```python
from build123d import *

# Parameters (mm, degrees)
F0_R     = 6
F1_DEPTH = 32
F3_W     = 12
F3_H     = 45
F4_DEPTH = 55.801
F5_R     = 4


with BuildPart() as f1:
    # F0 (on Front) → F1 (new body)
    with BuildSketch(Plane.XZ):
        with BuildLine():
            Line((15, -27.838539), (15, 58.161461))
            ThreePointArc((15, 58.161461), (-11.61895, 67.648294), (3, 43.464522))
            Line((3, 43.464522), (3, -27.838539))
            Line((3, -27.838539), (15, -27.838539))
        make_face()
        with Locations((0, 58.161461)):
            Circle(F0_R, mode=Mode.SUBTRACT)
    extrude(amount=F1_DEPTH)

    # F3 (on offset) → F4 (cut, through all)
    with BuildSketch(Plane.YZ.offset(-40.8)):
        with BuildLine():
            Line((0, -27.838539), (0, -11.838539))
            ThreePointArc((0, -11.838539), (-4.686292, -23.152248), (-16, -27.838539))
            Line((-16, -27.838539), (0, -27.838539))
        make_face()
        with BuildLine():
            Line((-32, -27.838539), (-16, -27.838539))
            ThreePointArc((-16, -27.838539), (-27.313708, -23.152248), (-32, -11.838539))
            Line((-32, -11.838539), (-32, -27.838539))
        make_face()
        with BuildLine():
            Line((-10, -11.838539), (-10, 13.161461))
            ThreePointArc((-10, 13.161461), (-16, 19.161461), (-22, 13.161461))
            Line((-22, 13.161461), (-22, -11.838539))
            ThreePointArc((-22, -11.838539), (-16, -17.838539), (-10, -11.838539))
        make_face()
        with Locations((-16, 50.661461)):
            Rectangle(F3_W, F3_H)
    extrude(amount=F4_DEPTH, mode=Mode.SUBTRACT)

    # F5
    f5_edges = [f1.edges().sort_by_distance(p)[0] for p in [
        (3, -5, 43.464522),
        (3, -27, 43.464522),
    ]]
    fillet(f5_edges, radius=F5_R)


solid = f1.part
```
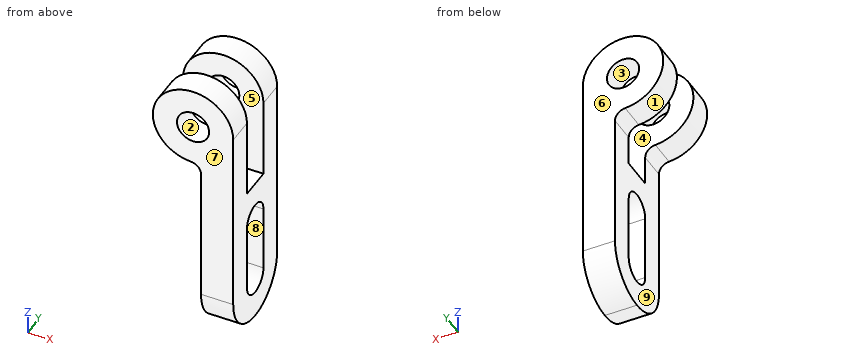
Can you work these out from the model? Positions are in its coordinate system, mm. Face numbers are marked on the shaded views. A direction names the side the tool comes from. Coordinates: 2 decimals unless noted, no trailing zeros. Write each loop counter-clockwise with the first axis right and the second up, starting at its lowest first coordinate (ties: lowest second). Pieces come first, ordered by that corner, then holes. Notation, with made-up numbers: M 86,-34 L 144,-34 A12 ccw 144,-28 Z; hole C -2.75,36.25 d6. An arc over 180 degrees is marked long. Write item = value, one per line. Start each with the question number.
Q1. If I drill on L1, parallel to Y at x = 2.5, z = 44; L2, parallel to X at y = -29, z = 1; L3, parallel to Z at x = 0, y = -2.5, over which ranges is the centre line in solid material (lowest first)? Write a range as [from, to].
Q2. If we section it at B-B, the plane y = -13.5: Write out the boundary of the cut face in (x, z), then the cut area to 3 significant figures.
Q3. If we section it at D-D, the plane y = -26: Write out the boundary of the cut face in (x, z).
Q4. On a 3-axis mill with a long thin cutter (end or side, diameter ignored), from which of +Z, -Z, +X, -X, +Y, -Y can I reach the whole of each face in a straight line? I mean the marked faces 5, 6, 7, 8 and 9. Say none if no direction works.
Q5. Thinking about a two-plate mould opening in X: for the marked faces 1, 2, 3 and 4, which applies, released by +X, released by -X, zero draft, split by the parting line, or undercut?
Q6. If we section it at C-C, the plane x = 8.5: Write out the boundary of the cut face in (y, z).
Q7. I'm going to push flat-ended pins straight in: pin 1 (13 mm diameter, centred on x = 7, y = -18, fed in from +Z); pin 2 (6 mm diameter, centred on y = -22, z = 31, fed in from -X); pin 3 (15 mm diameter, centred on x = -2.5, z = 55, fed in from +Y); pin 4 (8 mm diameter, centred on x = 7, y = -4.5, fed in from +Z). Where does each tip first touch, or does it pass through?
Q8. If we section it at A-A, the plane z = 31.5: Write out the boundary of the cut face in (x, y), then the cut area to 3 significant figures.
Check sheet entries:
q1.L1 = [-32, -22], [-10, 0]
q1.L2 = [3, 15]
q1.L3 = [43.06, 52.16], [64.16, 73.16]
q2.outline = M 3,-27.64 L 15,-27.64 L 15,-17.29 L 3,-17.29 Z; M 3,18.62 L 15,18.62 L 15,28.16 L 3,28.16 Z
q2.area = 239 mm²
q3.outline = M -0.79,43.18 A4 cw 3,39.19 L 3,-24.33 L 15,-24.33 L 15,58.16 A15 ccw long Z; hole C 0,58.16 d12
q4.face_5 = +Z, +X, -X
q4.face_6 = +Z, -Z, +X, -X, +Y
q4.face_7 = +Z, -Z, +X, -X, -Y
q4.face_8 = +X, -X
q4.face_9 = -Z, -X, +Y, -Y
q5.face_1 = split by the parting line
q5.face_2 = undercut
q5.face_3 = undercut
q5.face_4 = zero draft
q6.outline = M -32,-11.84 A16 ccw 0,-11.84 L 0,70.52 L -10,70.52 L -10,28.16 L -22,28.16 L -22,70.52 L -32,70.52 Z; hole M -22,-11.84 A6 ccw -10,-11.84 L -10,13.16 A6 ccw -22,13.16 Z
q7.pin_1 = 73.04
q7.pin_2 = 3
q7.pin_3 = 0
q7.pin_4 = 72.86
q8.outline = M 3,-32 L 15,-32 L 15,-22 L 3,-22 Z; M 3,-10 L 15,-10 L 15,0 L 3,0 Z
q8.area = 240 mm²
